Autodesk Inventor part; units mm, degrees
ref_plane "XZ Plane" through (0, 0, 0) normal (0, 1, 0) x (-1, 0, 0)
sketch "Sketch1" plane through (0, 0, 0) normal (0, 1, 0) x (-1, 0, 0)
  circle A0 centre (0, 0) radius 4
  dimension "d0" = 8
extrude "Extrusion1" add sketch "Sketch1" along normal blind 1
sketch "Sketch2" plane through (0, 1, 0) normal (0, 1, 0) x (1, 0, 0)
  circle A0 centre (0, 0) radius 4
  circle A1 centre (0, 0) radius 3
  dimension "d3" = 6
extrude "Extrusion2" add sketch "Sketch2" along normal blind 15.584 contours A1
sketch "Sketch3" plane through (0, 0, 0) normal (0, -1, 0) x (1, 0, 0)
  circle A0 centre (0, 0) radius 4
  circle A1 centre (0, 0) radius 1
  dimension "d6" = 2
extrude "Extrusion3" cut sketch "Sketch3" against normal blind 21 contours A1
sketch "Sketch4" plane through (0, 0, 0) normal (1, 0, 0) x (0, 1, 0)
  line L0 (1, 3) -> (16.584, 3)
  line L1 (1, -3) -> (16.584, -3)
  line L2 (0, 0) -> (17, 0)
  line L3 (16.584, 3) -> (18.8915, 0.25)
  line L4 (16.584, -3) -> (16.584, 3)
  line L5 (16.584, 0.2) -> (18.8915, 0.2)
  line L6 (17.7964, 0.3) -> (16.584, 1)
  line L7 (0, 1) -> (16.584, 1)
  line L8 (16.584, 1) -> (16.584, 3)
  line L9 (18.8915, 0.25) -> (18.8915, 0.2)
  line L10 (17.7964, 0.3) -> (19.4152, 0.3)
  line L11 (18.8076, 0.3) -> (18.8076, 0.35)
  point P0 (17.8856, 0.2)
  dimension "d9" = 40
  dimension "d10" = 0.2
  dimension "d11" = 30
  dimension "d20" = 0.05
  dimension "d21" = 0.3
  dimension "d22" = 0.05
revolve "Revolution1" add sketch "Sketch4" angle 360 about axis through (0, 0, 0) along (0, 1, 0) contours L3 L11 L10 L6 L4
sketch "Sketch5" plane through (0, 0, 0) normal (0, 0, 1) x (1, 0, 0)
  circle A0 centre (3, 1.35) radius 0.35
  line L0 (4, 1) -> (-4, 1)
  line L1 (3, 3) -> (3, 0)
  line L2 (0, 1.1204) -> (0, 3)
  line L3 (2.7525, 1.5975) -> (3.3734, 2.2184)
  line L4 (3.3734, 2.2184) -> (3.3499, 1.3406)
  point P0 (0, 0)
  dimension "d14" = 0.7
  dimension "d19" = 45
revolve "Revolution2" cut sketch "Sketch5" angle 360 about axis through (0, 1.1204, 0) along (0, 1, 0)
chamfer "Chamfer1" distance 0.3 angle 45 1 edges at (4, 1, 0)
sketch "Sketch6" plane through (0, 0, 0) normal (0, 0, 1) x (1, 0, 0)
  line L0 (-3, 1.845) -> (-3, 16.584)
  line L1 (-3, 3) -> (-2.4, 3)
  line L2 (-2.4, 3) -> (-2.4, 4)
  line L3 (-2.4, 4) -> (-3, 4)
  line L4 (-3, 4) -> (-3, 3)
  line L5 (-4, 0) -> (4, 0)
  line L6 (0, -3.7615) -> (0, 22.5691)
  point P0 (0, 0)
  dimension "d23" = 0.6
  dimension "d24" = 1
  dimension "d25" = 3
revolve "Revolution3" cut sketch "Sketch6" angle 360 about axis through (0, -10, 0) along (0, 1, 0)
properties part number "nozzle0.6" material "Copper"
Part model, mm, in its own coordinate system. A direction names the side the tool comes from. Coordinates: 2 decimals unless noted, no trailing zeros. Loops run counter-clockwise (first coordinate to the right, second up) from the corner with the lowest first, then second, coordinate; pieces in that order, holes last. Notation, with made-up numbers: (-7.5, 2.25) - (44.5, 2.25) arc R17 ccw to (44.5, 8.25) - close; hole circle Ø7 at (1, -18.75). An arc over 180 degrees is marked (long way). Write item = value, one per line. Start each with the question number.
Item 1: Cut at C-C, the plane y = 10. Give the cut face in (x, z).
Item 2: Cut at D-D, the plane y = 1.25. Give the cut face in (x, z), and give its area (3 significant figures).
Item 3: Wall check: L1, parallel to Z at x = 0, y = 12.25; L2, parallel to Y at x = 0.5, z = -2.5. Give the ranges that are in metal, low to high. Write a range as from..to.
Item 4: 3-axis set-ups, long thin cutter, end or side, ignore diameter. For faces 4 (the flat face through (1, 1, 3)), 5 (the cylindrical face through (-1.29, 3.507, 2.024)), 6 (the cylindrical face through (0, 8, -1)): which of +Z, -Z, +X, -X, +Y, -Y reach the whole face in a straight line?
Item 5: Flat gauge pins, fed straight in: pin 1 Ø1.5 at (x, y) = (-2.5, 14) entering from -Z; pin 2 Ø1.5 at (x, z) = (0.5, 3) entering from +Y; pin 3 Ø3 at (x, y) = (-2, 4) entering from -Z; pin 4 Ø3 at (x, z) = (0, 0) entering from +Y. Where does each tip first touch, or does it go through?
Item 6: Mould opens along X. For faces 1 (the conical face through (0.79, 18.42, -0.18)), 2 (the flat face through (-1, 0, -1)), 3 (the conical face through (0.3, 17.45, -0.4)) say: released by +X, released by -X, zero draft, split by the parting line, or undercut.
The answers:
q1.outline = circle Ø6 at (0, 0); hole circle Ø2 at (0, 0)
q2.outline = circle Ø5.33 at (0, 0); hole circle Ø2 at (0, 0)
q2.area = 19.2 mm2
q3.L1 = -3..-1, 1..3
q3.L2 = 0..3, 4..16.96
q4.face_4 = +Y
q4.face_5 = none
q4.face_6 = -Y
q5.pin_1 = -2.44
q5.pin_2 = 17.18
q5.pin_3 = -2.96
q5.pin_4 = 18.81
q6.face_1 = split by the parting line
q6.face_2 = zero draft
q6.face_3 = undercut
